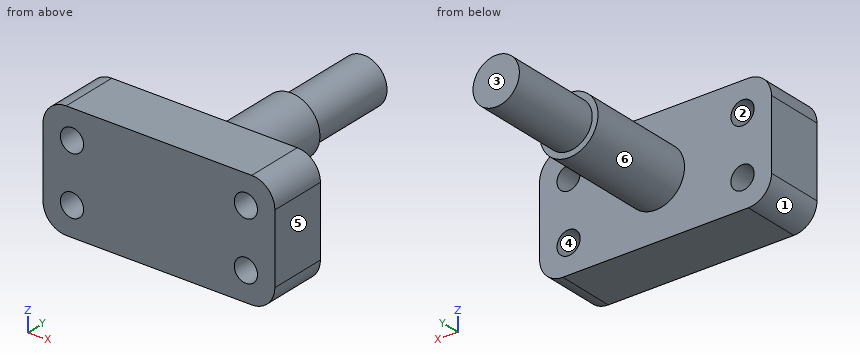
```python
from build123d import *

# Parameters (mm, degrees)
SKETCH1_R           = 2
BOSS_EXTRUDE1_DEPTH = 10
SKETCH2_R           = 5
BOSS_EXTRUDE2_DEPTH = 19
SKETCH3_R           = 4
BOSS_EXTRUDE3_DEPTH = 16


with BuildPart() as part:
    # Sketch1 → Boss-Extrude1 (new body)
    with BuildSketch(Plane(origin=(0, 0, 0), x_dir=(1, 0, 0), z_dir=(0, 1, 0))):
        with BuildLine():
            Line((4, 0), (36, 0))
            ThreePointArc((36, 0), (38.828427125, 1.171572875), (40, 4))
            Line((40, 4), (40, 16))
            ThreePointArc((40, 16), (38.828427125, 18.828427125), (36, 20))
            Line((36, 20), (4, 20))
            ThreePointArc((4, 20), (1.171572875, 18.828427125), (0, 16))
            Line((0, 16), (0, 4))
            ThreePointArc((0, 4), (1.171572875, 1.171572875), (4, 0))
        make_face()
        with Locations((5, 15)):
            Circle(SKETCH1_R, mode=Mode.SUBTRACT)
        with Locations((5, 5)):
            Circle(SKETCH1_R, mode=Mode.SUBTRACT)
        with Locations((35, 5)):
            Circle(SKETCH1_R, mode=Mode.SUBTRACT)
        with Locations((35, 15)):
            Circle(SKETCH1_R, mode=Mode.SUBTRACT)
    extrude(amount=BOSS_EXTRUDE1_DEPTH)

    # Sketch2 → Boss-Extrude2 (add)
    with BuildSketch(Plane(origin=(0, 10, 0), x_dir=(1, 0, 0), z_dir=(0, 1, 0))):
        with Locations((20, 10)):
            Circle(SKETCH2_R)
    extrude(amount=BOSS_EXTRUDE2_DEPTH)

    # Sketch3 → Boss-Extrude3 (add)
    with BuildSketch(Plane(origin=(0, 29, 0), x_dir=(1, 0, 0), z_dir=(0, 1, 0))):
        with Locations((20, 10)):
            Circle(SKETCH3_R)
    extrude(amount=BOSS_EXTRUDE3_DEPTH)


solid = part.part
```
Input: part model. Units: mm. Frame: model coordinates. Face numbers are marked on the shaded views. A direction names the side the tool comes from. Give positions to 0.01 mm unless a question says otherwise; leave off trailing zeros. Loops run counter-clockwise (first coordinate to the right, second up) from the corner with the lowest first, then second, coordinate; pieces in that order, holes last. Notation, with made-up numbers: M 87,-33.75 L 127,-33.75 A18 cw 127,-0.75 Z; hole C -16.75,26.5 d5. An arc over 180 degrees is marked long. Answer as CSV lines item,"result". Start each with the question number.
1. Section D-D on x = 20. Return loops of the section in (y, z).
2. Section C-C on y = 3.5. Return loops of the section in (x, z).
3. Reachability of the marked faces 5 and 6 from +Z, -Z, +X, -X, +Y, -Y: full face, straight path, thin tool, end or side. Return the list, or none.
4. Pin query (flat end, axial travel): P1, Ø4, axis at y = 30.5, z = -14.5, coming from the -X side; P2, Ø5, axis at x = 35, z = -15, coming from the +Y side; P3, Ø3, axis at y = 13.5, z = -10, coming from the -X side. Return the tip coordinate at first contact, or that it passes through.
5. Section B-B on z = -10. Return loops of the section in (x, y).
6. Pull-direction query (X, two-part tool) for the marked faces 1, 2, 3 and 4; classes: released by +X, released by -X, zero draft, split by the parting line, or undercut.
7. Line query: L1, parallel to Z at x = 35, y = 7; L2, parallel to X at y = 6.5, z = -5; L3, parallel to Y at x = 26, z = -12. Output: solid intervals per line, ascending.
8. Section A-A on x = 35. Return loops of the section in (y, z), plus the area to 3 significant figures.
Computed values:
1,outline,"M 0,-20 L 10,-20 L 10,-15 L 29,-15 L 29,-14 L 45,-14 L 45,-6 L 29,-6 L 29,-5 L 10,-5 L 10,0 L 0,0 Z"
2,outline,"M 0,-16 A4 ccw 4,-20 L 36,-20 A4 ccw 40,-16 L 40,-4 A4 ccw 36,0 L 4,0 A4 ccw 0,-4 Z; hole C 5,-15 d4; hole C 5,-5 d4; hole C 35,-15 d4; hole C 35,-5 d4"
3,face 5,"+Z, -Z, +X, +Y, -Y"
3,face 6,"+Y"
4,P1,"stops at x = 16.14"
4,P2,"stops at y = 10"
4,P3,"stops at x = 15"
5,outline,"M 0,0 L 40,0 L 40,10 L 25,10 L 25,29 L 24,29 L 24,45 L 16,45 L 16,29 L 15,29 L 15,10 L 0,10 Z"
6,face 1,"released by -X"
6,face 2,"undercut"
6,face 3,"zero draft"
6,face 4,"undercut"
7,L1,"z = -20 to -17, -13 to -7, -3 to 0"
7,L2,"x = 0 to 3, 7 to 33, 37 to 40"
7,L3,"y = 0 to 10"
8,outline,"M 0,-20 L 10,-20 L 10,-17 L 0,-17 Z; M 0,-13 L 10,-13 L 10,-7 L 0,-7 Z; M 0,-3 L 10,-3 L 10,0 L 0,0 Z"
8,area,"120 mm²"
